from build123d import *

# Parameters (mm, degrees)
F0_R     = 3.75
F0_W     = 15
F0_H     = 10
F1_DEPTH = 35
F3_DEPTH = 60.001
F4_W     = 20
F4_H     = 5
F5_DEPTH = 100.001


with BuildPart() as f1:
    # F0 (on Top) → F1 (new body)
    with BuildSketch(Plane.XY):
        Polygon((50, 25), (-50, 25), (-50, -25), (0, -25), (15, -25), (50, -25), align=None)
        with Locations((17.5, -12.5)):
            Circle(F0_R, mode=Mode.SUBTRACT)
        with Locations((37.5, -12.5)):
            Circle(F0_R, mode=Mode.SUBTRACT)
        with Locations((17.5, 12.5)):
            Circle(F0_R, mode=Mode.SUBTRACT)
        with Locations((37.5, 12.5)):
            Circle(F0_R, mode=Mode.SUBTRACT)
        with Locations((7.5, -30)):
            Rectangle(F0_W, F0_H)
    extrude(amount=F1_DEPTH)

    # F2 (on face) → F3 (cut, through all)
    with BuildSketch(Plane(origin=(0, 25, 0), x_dir=(-1, 0, 0), z_dir=(0, 1, 0))):
        Polygon((-50, 35), (-50, 0), (0, 35), align=None)
    extrude(amount=-F3_DEPTH, mode=Mode.SUBTRACT)

    # F4 (on face) → F5 (cut, through all)
    with BuildSketch(Plane(origin=(-50, 0, 0), x_dir=(0, -1, 0), z_dir=(-1, 0, 0))):
        with Locations((0, 32.5)):
            Rectangle(F4_W, F4_H)
    extrude(amount=-F5_DEPTH, mode=Mode.SUBTRACT)


solid = f1.part
Verification items for the finished model (mm, model axes). A direction names the side the tool comes from. Coordinates: 2 decimals unless noted, no trailing zeros. Write each loop counter-clockwise with the first axis right and the second up, starting at its lowest first coordinate (ties: lowest second). Pieces come first, ordered by that corner, then holes. Notation, with made-up numbers: (84.5, -5.5) -> (92.5, -5.5) arc R25 ccw to (92.5, 11.5) -> close; hole circle Ø7 at (7, 1.5). An arc over 180 degrees is marked (long way). One line per item, written item: value. Start each with the question number.
Q1. Cross-section at A-A on x = 37.5. Enter the section's corners in (y, z), and give its area (3 significant figures).
Q2. Go/stop test with flat-tipped pins: P1, Ø2, axis at x = -11.5, y = -26.5, coming from the -Z side; P2, Ø1.5, axis at x = -16.5, z = 33, coming from the -Y side; P3, Ø4, axis at x = 25.5, y = 17, coming from the +Z side; P4, Ø12, axis at x = 17.5, y = -12.5, coming from the +Z side. Record where each tip stops, or that it passes through.
Q3. Cross-section at B-B on y = -12.5. Enter the section's corners in (x, z) (3 decimals).
Q4. Thickness scan on L1, parallel to Y at x = 17.5, z = 16.75; L2, parallel to X at y = -14, z = 3; L3, parallel to X at y = 12.5, z = 18.25. Record the ranges inside material, lowest first. Write a range as from..to.
Q5. Cross-section at D-D on z = 31. Enter the section's corners in (x, y), and give its area (3 significant figures).
Q6. Mould release check, pull along Y, two halves, no side actions. Record for faces 6 (the cylindrical face through (33.754, -12.335, 4.386)), 7 (the flat face through (0, -30, 17)), 8 (the flat face through (-10, 25, 17)): pulls with the +Y half, pulls with the -Y half, needs draft (parallel to the pull), parting line crosses it, or undercut.
Q7. Access from +Z, -Z, +X, -X, +Y, -Y to the whole of each face (thin tool, end or side, straight path). Record for faces 1 (the flat face through (-1, -5, 0)), 2 (the flat face through (-25, -25, 17)), 3 (the cylindrical face through (33.754, 12.665, 4.386)), 4 (the flat face through (15, -30, 12)), 5 (the flat face through (-22, 0, 30)).
Q8. Cross-section at C-C on z = 18.5. Enter the section's corners in (x, y).
Checked values:
1. outline: (-25, 0) -> (-16.25, 0) -> (-16.25, 8.75) -> (-25, 8.75) -> close; (-8.75, 0) -> (8.75, 0) -> (8.75, 8.75) -> (-8.75, 8.75) -> close; (16.25, 0) -> (25, 0) -> (25, 8.75) -> (16.25, 8.75) -> close
1. area: 306 mm²
2. P1: passes through
2. P2: stops at y = -25
2. P3: stops at z = 18.55
2. P4: stops at z = 26.95
3. outline: (-50, 0) -> (13.75, 0) -> (13.75, 25.375) -> (0, 35) -> (-50, 35) -> close; (21.25, 0) -> (33.75, 0) -> (33.75, 11.375) -> (21.25, 20.125) -> close; (41.25, 0) -> (50, 0) -> (41.25, 6.125) -> close
4. L1: y = -25..-16.25, -8.75..8.75, 16.25..25
4. L2: x = -50..14.06, 20.94..34.06, 40.94..45.71
4. L3: x = -50..13.75, 21.25..23.93
5. outline: (-50, -25) -> (0, -25) -> (0, -35) -> (5.71, -35) -> (5.71, -10) -> (-50, -10) -> close; (-50, 10) -> (5.71, 10) -> (5.71, 25) -> (-50, 25) -> close
5. area: 1,730 mm²
6. face 6: undercut
6. face 7: needs draft
6. face 8: pulls with the +Y half
7. face 1: -Z, +X, -X, +Y, -Y
7. face 2: +Z, -Z, -X, -Y
7. face 3: +Z, -Z
7. face 4: +Z, -Z, +X, -Y
7. face 5: +Z, +X, -X
8. outline: (-50, -25) -> (0, -25) -> (0, -35) -> (15, -35) -> (15, -25) -> (23.57, -25) -> (23.57, 25) -> (-50, 25) -> close; hole circle Ø7.5 at (17.5, -12.5); hole circle Ø7.5 at (17.5, 12.5)
